The listing builds one solid part. Answer for the finished solid, in the listing's coordinates (mm). A direction names the side the tool comes from. Give positions to 0.01 mm unless a question says otherwise; leave off trailing zeros. Order: outer loops, then holes, each group sorted by start corner. A loop starts at its lowest first (then second) coordinate and runs counter-clockwise, first axis right, second up.
```python
from build123d import *

# Parameters (mm, degrees)
SKETCH1_W           = 800
SKETCH1_H           = 400
BOSS_EXTRUDE1_DEPTH = 50
FILLET1_R           = 60
SKETCH3_W           = 68.405794472
SKETCH3_H           = 72.041840608
BOSS_EXTRUDE2_DEPTH = 30
SKETCH5_W           = 68
SKETCH5_H           = 72
BOSS_EXTRUDE3_DEPTH = 9


with BuildPart() as part:
    # Sketch1 → Boss-Extrude1 (new body)
    with BuildSketch(Plane(origin=(0, 0, 0), x_dir=(1, 0, 0), z_dir=(0, 1, 0))):
        Rectangle(SKETCH1_W, SKETCH1_H)
    extrude(amount=BOSS_EXTRUDE1_DEPTH)

    # Fillet1
    fillet1_edges = [part.edges().sort_by_distance(p)[0] for p in [
        (400, 25, 200),
        (-400, 25, 200),
        (-400, 25, -200),
        (400, 25, -200),
    ]]
    fillet(fillet1_edges, radius=FILLET1_R)

    # Sketch3 → Boss-Extrude2 (add)
    with BuildSketch(Plane(origin=(0, 50, 0), x_dir=(1, 0, 0), z_dir=(0, 1, 0))):
        with Locations((-300, 0)):
            Rectangle(SKETCH3_W, SKETCH3_H)
    extrude(amount=BOSS_EXTRUDE2_DEPTH)

    # Sketch5 → Boss-Extrude3 (add)
    with BuildSketch(Plane(origin=(0, 50, 0), x_dir=(1, 0, 0), z_dir=(0, 1, 0))):
        with Locations((330, 0)):
            Rectangle(SKETCH5_W, SKETCH5_H)
    extrude(amount=BOSS_EXTRUDE3_DEPTH)


solid = part.part
```
1) Straight lines are drawn through the part: probe 1 along Y at (x, z) = (4.5, 2); probe 2 along X at (y, z) = (27, -142); probe 3 along X at (y, z) = (21, -182). For each, find the intervals that lie inside material, in ascending order.
Geometry says:
probe 1: y = 0 to 50
probe 2: x = -399.97 to 399.97
probe 3: x = -382.85 to 382.85
2) Find section A-A (z = 13.5). Write down the section's boundary in (x, y).
Geometry says:
outline: (-400, 0) - (400, 0) - (400, 50) - (364, 50) - (364, 59) - (296, 59) - (296, 50) - (-265.8, 50) - (-265.8, 80) - (-334.2, 80) - (-334.2, 50) - (-400, 50) - close
3) Given P1, Ø7, axis at x = 337.5, y = 54.5, coming from the +Z side; P2, Ø2.5, axis at y = 56, z = -1, coming from the +X side; P3, Ø3, axis at x = 262, z = 87.5, coming from the +Y side, each flat-ended and moving along its own axis, determine where each tip first touches the part or whether it passes through.
Geometry says:
P1: stops at z = 36
P2: stops at x = 364
P3: stops at y = 50
4) Find section D-D (z = 105). Write down the section's boundary in (x, y).
Geometry says:
outline: (-400, 0) - (400, 0) - (400, 50) - (-400, 50) - close
5) Find section C-C (x = 170). Write down the section's boundary in (y, z), then the cut area to 3 significant figures.
Geometry says:
outline: (0, -200) - (50, -200) - (50, 200) - (0, 200) - close
area: 20,000 mm2
6) For a pull along X with two mould halves and no side action, classify faces 4 (the cylindrical face through (-382.89, 25.35, 181.96)), 5 (the flat face through (-5, 25, -200)), 6 (the flat face through (-265.797, 65, 1)) as +X half, -X half, draft (parallel to the pull), parting line (faces both ways), or undercut.
Geometry says:
face 4: -X half
face 5: draft
face 6: undercut
7) Find section B-B (x = -309). Write down the section's boundary in (y, z), then the cut area to 3 significant figures.
Geometry says:
outline: (0, -200) - (50, -200) - (50, -36.02) - (80, -36.02) - (80, 36.02) - (50, 36.02) - (50, 200) - (0, 200) - close
area: 22,200 mm2
8) A tool of negligible diameter and unlimited length cuts with its end or side. For faces 1 (the flat face through (-334.203, 65, 1)), 2 (the flat face through (-300, 65, 36.021)), 3 (the flat face through (-300, 65, -36.021)), from which of +Z, -Z, +X, -X, +Y, -Y can it reach the whole face along a straight path? Write none if from no direction.
Geometry says:
face 1: +Z, -Z, -X, +Y
face 2: +Z, +X, -X, +Y
face 3: -Z, +X, -X, +Y
